Job drawing, mm, ordinate dimensions from the low corner. One solid piece. A direction names the side the tool comes from. Coordinates: 2 decimals unless noted, no trailing zeros. Write each loop counter-clockwise with the first axis right and the second up, starting at its lowest first coordinate (ties: lowest second). Pieces come first, ordered by that corner, then holes. Notation, with made-up numbers: (66.5, 11) - (103.5, 11) arc R21 ccw to (103.5, 26) - close; hole circle Ø5 at (-32, 49.5). An arc over 180 degrees is marked (long way). Use a Markdown table: item, result.
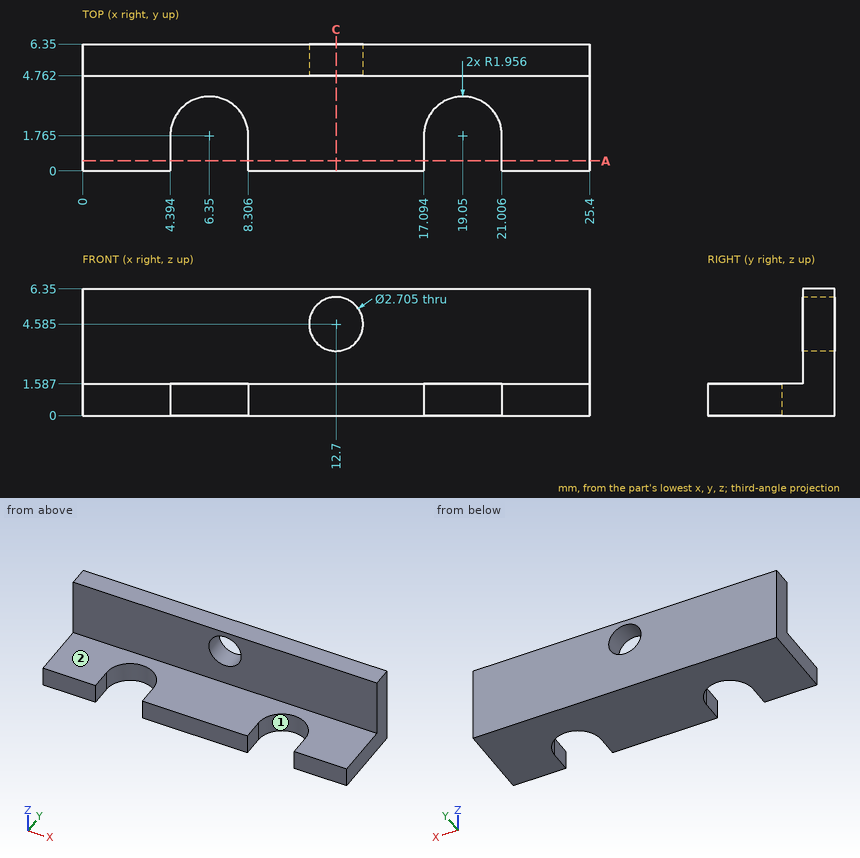
Item 1: Drill centre lines: probe 1 along Z at (x, y) = (12.7, 5.9); probe 2 along Y at (x, z) = (22.5, 4); probe 3 along Z at (x, y) = (12.25, 3.75). Where is each one in solid material? Low to high.
From the geometry:
| item | result |
|---|---|
| probe 1 | 0 to 3.23, 5.94 to 6.35 |
| probe 2 | 4.76 to 6.35 |
| probe 3 | 0 to 1.59 |
Item 2: Which spindle directions (+Z, -Z, +X, -X, +Y, -Y) get a long thin tool onto all of the face, cutting with end or side? Do the marked faces 1 and 2. Say none if no direction does.
From the geometry:
| item | result |
|---|---|
| face 1 | +Z, -Z, -Y |
| face 2 | +Z, +X, -X, -Y |
Item 3: Band-saw the part on A-A, the plane y = 0.5. Give the cut face in (x, z) (1 decimal), then the cut area to 3 significant figures.
From the geometry:
| item | result |
|---|---|
| outline | (0, 0) - (4.4, 0) - (4.4, 1.6) - (0, 1.6) - close; (8.3, 0) - (17.1, 0) - (17.1, 1.6) - (8.3, 1.6) - close; (21, 0) - (25.4, 0) - (25.4, 1.6) - (21, 1.6) - close |
| area | 27.9 mm^2 |
Item 4: Band-saw the part on C-C, the plane x = 12.7. Give the cut face in (y, z).
From the geometry:
| item | result |
|---|---|
| outline | (0, 0) - (6.35, 0) - (6.35, 3.23) - (4.76, 3.23) - (4.76, 1.59) - (0, 1.59) - close; (4.76, 5.94) - (6.35, 5.94) - (6.35, 6.35) - (4.76, 6.35) - close |
Item 5: Drop a flat-ended pin along its axis: P1, Ø3.5, axis at x = 12.7, z = 4.58, coming from the -Y side. Give the stop position or say it passes through.
From the geometry:
| item | result |
|---|---|
| P1 | y = 4.76 |
